Design review of the part built by this model. Coordinates are the model's own, in mm. A direction names the side the tool comes from. Round coordinates to 2 decimals unless told otherwise and drop trailing zeros. Write each loop counter-clockwise with the first axis right and the second up, starting at its lowest first coordinate (ties: lowest second). Pieces come first, ordered by that corner, then holes. Notation, with made-up numbers: M -7.5,-10.5 L -3.5,-10.5 A14 ccw -3.5,10.5 Z; hole C 58.25,73 d8. An arc over 180 degrees is marked long. One line per question, with ' | ' between items. Start each with the question number.
Item 1: For L1, parallel to Y at x = -1, z = -62; L2, parallel to X at y = 2.25, z = -90.5; L3, parallel to Y at x = -8, z = -80, list the stretches that pass through material, from the lowest coordinate up.
Item 2: Insertion check: pin 1 Ø4 at (y, z) = (5.5, -28) entering from +X; pin 2 Ø6 at (x, z) = (5, -108.5) entering from -Y; pin 3 Ø6 at (x, z) = (0, -40) entering from +Y. Each pin has a flat end and moves straight along its axis. Give the tip position at first contact, or say it passes through.
Item 3: Draft analysis for pull direction Z (two halves, no side actions). For faces 1 (the face through (6.466, 2.681, -35.962)), 2 (the face through (-1.38, 6.23, -3.22)), 3 (the face through (-2, -5, -24.5)), state which applies: released by +Z, released by -Z, zero draft, split by the parting line, or undercut.
Item 4: Machinability: for faces 4 (the face through (2, -5, -18)), 5 (the face through (6.466, 2.681, -12.575)), 6 (the face through (0, 0, 0)), which of the approach directions +Z, -Z, +X, -X, +Y, -Y give a long, thin tool a straight path to every point of the face, cutting with its end or side? Answer none if there is none.
Item 5: Add section A-A, the plane z = -104. State the section outline as (x, y) points, and give its area (3 significant figures).
```python
from build123d import *


with BuildPart() as part:
    # Sketch1 → Revolve1 (revolve)
    with BuildSketch(Plane(origin=(0, 0, 0), x_dir=(1, 0, 0), z_dir=(0, 1, 0))):
        with BuildLine():
            Line((0, 0), (0, 148.5))
            ThreePointArc((0, 148.5), (8.909545443, 144.809545443), (12.6, 135.9))
            Line((12.6, 135.9), (12.6, 75.9))
            ThreePointArc((12.6, 75.9), (11.674574623, 66.505013574), (8.93386968, 57.471148483))
            ThreePointArc((8.93386968, 57.471148483), (7.488158337, 52.705819301), (7, 47.75))
            Line((7, 47.75), (7, 24.5))
            Line((7, 24.5), (5, 24.5))
            Line((5, 24.5), (5, 18))
            Line((5, 18), (7, 18))
            Line((7, 18), (7, 7.3))
            Line((7, 7.3), (6.15, 1.7))
            Line((6.15, 1.7), (5, 1.7))
            Line((5, 1.7), (5, 0))
            Line((5, 0), (0, 0))
        make_face()
    revolve(axis=Axis((0, 0, 0), (0, 0, -1)))


solid = part.part
```
Computed values:
1) L1: y = -10.5 to 10.5 | L2: x = -12.4 to 12.4 | L3: y = -9.73 to 9.73
2) pin 1: stops at x = 6.06 | pin 2: stops at y = -12.44 | pin 3: stops at y = 7
3) face 1: zero draft | face 2: released by +Z | face 3: undercut
4) face 4: none | face 5: +Z | face 6: +Z, +X, -X, +Y, -Y
5) outline: C 0,0 d25.2 | area: 499 mm^2
